from build123d import *

# Parameters (mm, degrees)
SKETCH001_W   = 3
SKETCH001_H   = 0.5
SKETCH001_W_2 = 2
SKETCH001_W_3 = 0.5
SKETCH001_H_2 = 2
PAD_DEPTH     = 5
SKETCH002_R   = 2
POCKET_DEPTH  = 12
CHAMFER_SIZE  = 0.5


with BuildPart() as part:
    # Sketch → Revolution (revolve)
    with BuildSketch(Plane.XZ):
        Polygon((0, 0), (0, 4.9), (2, 4.9), (2, 4), (16, 4), (16, 0), align=None)
    revolve(axis=Axis((0, 0, 0), (1, 0, 0)))

    # Sketch001 → Pad (new body)
    with BuildSketch(Plane.YZ.offset(16)):
        with Locations((0, -3)):
            Rectangle(SKETCH001_W, SKETCH001_H)
        with Locations((0, 3)):
            Rectangle(SKETCH001_W_2, SKETCH001_H)
        with Locations((3, 0)):
            Rectangle(SKETCH001_W_3, SKETCH001_H_2)
        with Locations((-3, 0)):
            Rectangle(SKETCH001_W_3, SKETCH001_H_2)
    extrude(amount=PAD_DEPTH)

    # Sketch002 → Pocket (cut)
    with BuildSketch(Plane.YZ):
        Circle(SKETCH002_R)
    extrude(amount=POCKET_DEPTH, mode=Mode.SUBTRACT)

    # Chamfer
    chamfer_edges = [part.edges().sort_by_distance(p)[0] for p in [
        (0, 0, -4.9),
        (0, -2, 0),
    ]]
    chamfer(chamfer_edges, length=CHAMFER_SIZE)


solid = part.part
Geometry check sheet. Reference: the model listing, model coordinates, mm. A direction names the side the tool comes from. Round coordinates to 2 decimals unless told otherwise and drop trailing zeros. Order: outer loops, then holes, each group sorted by start corner. A loop starts at its lowest first (then second) coordinate and runs counter-clockwise, first axis right, second up. Notation, with made-up numbers: M 54.25,63.25 L 70.25,63.25 A22 ccw 70.25,72.25 Z; hole C 2.5,-37.75 d6. An arc over 180 degrees is marked long. Answer in a Markdown table with one row per item. Add a question column.
Item 1: Sectioned sample at B-B, the plane z = 0. Enter the section's corners in (x, y).
Item 2: Depth check by flat-ended pin: pin 1 Ø3.5 at (x, y) = (18.5, 0.5) entering from -Z; pin 2 Ø1 at (x, z) = (18, -0.5) entering from +Y; pin 3 Ø0.6 at (x, z) = (18.5, 0) entering from -Y. Enter the tip coordinate at first touch or a pass-through.
Item 3: Draft check along Z on faces 5 (the face through (18, 0, 3.25)), 6 (the face through (9.098, 3.905, -0.867)), 7 (the face through (0, 2, -2)), 8 (the face through (18, 0, 2.75)). Enter one of: released by +Z, released by -Z, zero draft, split by the parting line, or undercut.
Item 4: Sectioned sample at A-A, the plane x = 17.5. Enter the section's corners in (y, z), plus the area to 3 significant figures.
Item 5: Material ranges on L1, parallel to Z at x = 5.75, y = 0; L2, parallel to Z at x = 17.75, y = -0.5; L3, parallel to X at y = 2.5, z = 1.75, recorded low to high. Write a range as [from, to].
Item 6: Set-up check for faces 1 (the face through (18, 3.25, 0)), 2 (the face through (18, -2.75, 0)), 3 (the face through (18, 0, -2.75)), 4 (the face through (18, 0, -3.25)): record each of +Z, -Z, +X, -X, +Y, -Y from which the full face is reachable in a straight line by a thin tool's end or side.
Item 7: Sectioned sample at D-D, the plane x = 13.75. Enter the section's corners in (y, z), plus the area to 3 significant figures.
Filled in:
| question | item | result |
|---|---|---|
| 1 | outline | M 0,-4.4 L 0.5,-4.9 L 2,-4.9 L 2,-4 L 16,-4 L 16,-3.25 L 21,-3.25 L 21,-2.75 L 16,-2.75 L 16,2.75 L 21,2.75 L 21,3.25 L 16,3.25 L 16,4 L 2,4 L 2,4.9 L 0.5,4.9 L 0,4.4 L 0,2.5 L 0.5,2 L 12,2 L 12,-2 L 0.5,-2 L 0,-2.5 Z |
| 2 | pin 1 | stops at z = -3.25 |
| 2 | pin 2 | stops at y = 3.25 |
| 2 | pin 3 | stops at y = -3.25 |
| 3 | face 5 | released by +Z |
| 3 | face 6 | split by the parting line |
| 3 | face 7 | zero draft |
| 3 | face 8 | undercut |
| 4 | outline | M -3.25,-1 L -2.75,-1 L -2.75,1 L -3.25,1 Z; M -1.5,-3.25 L 1.5,-3.25 L 1.5,-2.75 L -1.5,-2.75 Z; M -1,2.75 L 1,2.75 L 1,3.25 L -1,3.25 Z; M 2.75,-1 L 3.25,-1 L 3.25,1 L 2.75,1 Z |
| 4 | area | 4.50 mm² |
| 5 | L1 | z = [-4, -2], [2, 4] |
| 5 | L2 | z = [-3.25, -2.75], [2.75, 3.25] |
| 5 | L3 | x = [0, 16] |
| 6 | face 1 | +Z, -Z, +X, +Y |
| 6 | face 2 | +Z, -Z, +X |
| 6 | face 3 | +X, +Y, -Y |
| 6 | face 4 | -Z, +X, +Y, -Y |
| 7 | outline | C 0,0 d8 |
| 7 | area | 50.3 mm² |
